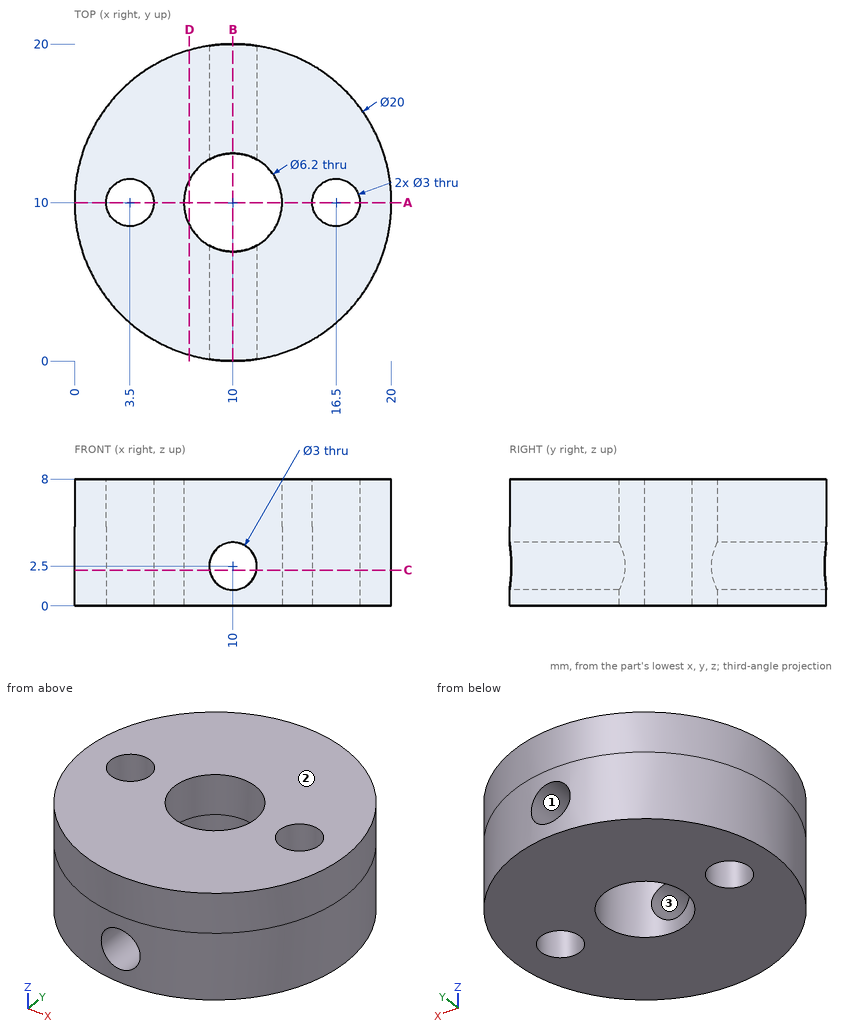
Design review of the part shown in the three views and the two pictorial views. Dimensions are in mm from the part's minimum x, y and z. Coordinates: 2 decimals unless noted, no trailing zeros. Loops run counter-clockwise (first coordinate to the right, second up) from the corner with the lowest first, then second, coordinate; pieces in that order, holes last. Notation, with made-up numbers: (68, 89) - (87, 89) arc R24 cw to (87, 124) - close; hole circle Ø1 at (54.5, 5). An arc over 180 degrees is marked (long way). Use a Markdown table: item, result. Add a question column.
Item 1: Mouldability with a two-part tool opening along X and no side actions: class the marked faces 1, 2 and 3 as pulls with the +X half, pulls with the -X half, needs draft (parallel to the pull), parting line crosses it, or undercut.
Item 2: We need section D-D (x = 7.25). Give the boundary of the cut face in (y, z), and give its area (3 significant figures).
Item 3: We need section A-A (y = 10). Give the boundary of the cut face in (x, z).
Item 4: For line 1 (Z direction, x = 10, y = 2.75); line 2 (Y direction, x = 4.75, z = 5.5); line 3 (X direction, y = 10.75, z = 1), list the stretches that pass through material, from the lowest coordinate up.
Item 5: We need section C-C (z = 2.25). Give the boundary of the cut face in (x, y), and give its area (3 significant figures).
Item 6: Insertion check: pin 1 Ø4 at (x, y) = (3.5, 10) entering from -Z; pin 2 Ø1.5 at (y, z) = (6.5, 2) entering from -X; pin 3 Ø3 at (y, z) = (12.5, 7) entering from -X. Each pin has a flat end and moves straight along its axis. Give the tip position at first contact, or say it passes through.
Item 7: We need section B-B (x = 10). Give the boundary of the cut face in (y, z).
Results list:
| question | item | result |
|---|---|---|
| 1 | face 1 | undercut |
| 1 | face 2 | needs draft |
| 1 | face 3 | undercut |
| 2 | outline | (0.39, 0) - (8.57, 0) - (8.57, 8) - (0.39, 8) - close; (11.43, 0) - (19.61, 0) - (19.61, 8) - (11.43, 8) - close |
| 2 | area | 131 mm^2 |
| 3 | outline | (0, 0) - (2, 0) - (2, 8) - (0, 8) - close; (5, 0) - (6.9, 0) - (6.9, 8) - (5, 8) - close; (13.1, 0) - (15, 0) - (15, 8) - (13.1, 8) - close; (18, 0) - (20, 0) - (20, 8) - (18, 8) - close |
| 4 | line 1 | z = 0 to 1, 4 to 8 |
| 4 | line 2 | y = 1.49 to 9.17, 10.83 to 18.51 |
| 4 | line 3 | x = 0.03 to 2.2, 4.8 to 6.99, 13.01 to 15.2, 17.8 to 19.97 |
| 5 | outline | (8.52, 0.11) - (8.52, 7.28) arc R3.1 cw to (8.52, 12.72) - (8.52, 19.89) arc R10 ccw to start; (11.48, 0.11) arc R10 ccw to (11.48, 19.89) - (11.48, 12.72) arc R3.1 cw to (11.48, 7.28) - close; hole circle Ø3 at (3.5, 10); hole circle Ø3 at (16.5, 10) |
| 5 | area | 229 mm^2 |
| 6 | pin 1 | stops at z = 0 |
| 6 | pin 2 | stops at x = 0.39 |
| 6 | pin 3 | stops at x = 0.05 |
| 7 | outline | (0, 0) - (6.9, 0) - (6.9, 1) - (0, 1) - close; (0, 4) - (6.9, 4) - (6.9, 8) - (0, 8) - close; (13.1, 0) - (20, 0) - (20, 1) - (13.1, 1) - close; (13.1, 4) - (20, 4) - (20, 8) - (13.1, 8) - close |
